Input: part model. Units: mm. Frame: model coordinates. A direction names the side the tool comes from. Round coordinates to 2 decimals unless told otherwise and drop trailing zeros. Loops run counter-clockwise (first coordinate to the right, second up) from the corner with the lowest first, then second, coordinate; pieces in that order, holes last. Notation, with made-up numbers: (42.5, 52.5) -> (65.5, 52.5) arc R15 cw to (65.5, 64.5) -> close; hole circle Ø3 at (26.25, 17.5). An arc over 180 degrees is marked (long way). Answer in a Markdown table with one row per item. Add a question column.
Q1. Section C-C, the plane x = -11. Output: boundary loops of the cut face in (y, z), and give its area (3 significant figures).
Q2. Section D-D, the plane x = -40.5. Output: boundary loops of the cut face in (y, z), and give its area (3 significant figures).
Q3. Section A-A, the plane x = 47.5. Output: boundary loops of the cut face in (y, z), and give its area (3 significant figures).
Q4. Pin query (flat end, axial travel): pin 1 (6.5 mm diameter, centred on x = -28.5, z = 2, fed in from +Y); pin 2 (2.5 mm diameter, centred on y = 4, z = -5, fed in from +X). Return the tip coordinate at first contact, or that it passes through.
Q5. Reachability of faces 1 (the face through (8.25, 4, 0)), 2 (the face through (57.79, 4.39, -6.24)), 3 (the face through (-1, 3, 10.5)), 4 (the face through (-58, 10, 0)), 5 (the face through (-1, 0, -7)) from +Z, -Z, +X, -X, +Y, -Y: full face, straight path, thin tool, end or side. Return the list, or none.
Q6. Mould query, pull axis Z, two halves, no side actions, for faces 6 (the face through (-39.774, 3.944, -2.433)), 7 (the face through (-11.479, 10.859, -9.297)), 8 (the face through (-43, 8, -7)). Classes: pulls with the +Z half, pulls with the -Z half, needs draft (parallel to the pull), parting line crosses it, or undercut.
Q7. Ray query, L1, parallel to X at y = 6.75, z = 0.25; L2, parallel to X at y = 8.5, z = -8.5; L3, parallel to Y at x = 55.25, z = -5. Return the intervals inside material, ascending. Write a range as from..to.
Q8. Section B-B, the plane y = 4. Give the number of separate pieces and of enclosed holes in the cut face, and give its area (3 significant figures).
```python
from build123d import *

# Parameters (mm, degrees)
SKETCH1_W           = 122
SKETCH1_H           = 21
SKETCH1_R           = 8.1
BOSS_EXTRUDE1_DEPTH = 8
CUT_EXTRUDE1_DEPTH  = 122
FILLET2_R           = 1
SKETCH6_W           = 3
SKETCH6_H           = 21
BOSS_EXTRUDE4_DEPTH = 4
FILLET3_R           = 4
SKETCH7_R           = 1.3
CUT_EXTRUDE2_DEPTH  = 10


with BuildPart() as part:
    # Sketch1 → Boss-Extrude1 (new body)
    with BuildSketch(Plane(origin=(0, 0, 0), x_dir=(1, 0, 0), z_dir=(0, 1, 0))):
        Rectangle(SKETCH1_W, SKETCH1_H)
        with Locations((-47.5, 0)):
            Circle(SKETCH1_R, mode=Mode.SUBTRACT)
        with Locations((-23.5, 0)):
            Circle(SKETCH1_R, mode=Mode.SUBTRACT)
        with Locations((23.5, 0)):
            Circle(SKETCH1_R, mode=Mode.SUBTRACT)
        with Locations((47.5, 0)):
            Circle(SKETCH1_R, mode=Mode.SUBTRACT)
    extrude(amount=BOSS_EXTRUDE1_DEPTH)

    # Sketch4 → Cut-Extrude1 (cut)
    with BuildSketch(Plane(origin=(0, 8, 0), x_dir=(1, 0, 0), z_dir=(0, 1, 0))):
        with BuildLine():
            Line((8.25, 4), (4.472135955, 4))
            ThreePointArc((4.472135955, 4), (5.605034154, 2.140932539), (6, 0))
            ThreePointArc((6, 0), (5.605034154, -2.140932539), (4.472135955, -4))
            Line((4.472135955, -4), (8.25, -4))
            Line((8.25, -4), (8.25, 4))
        make_face()
        with BuildLine():
            Line((4.472135955, 4), (-4.472135955, 4))
            ThreePointArc((-4.472135955, 4), (-6, 0), (-4.472135955, -4))
            Line((-4.472135955, -4), (4.472135955, -4))
            ThreePointArc((4.472135955, -4), (5.605034154, -2.140932539), (6, 0))
            ThreePointArc((6, 0), (5.605034154, 2.140932539), (4.472135955, 4))
        make_face()
        with BuildLine():
            ThreePointArc((4.472135955, 4), (0, 6), (-4.472135955, 4))
            Line((-4.472135955, 4), (4.472135955, 4))
        make_face()
        with BuildLine():
            Line((4.472135955, -4), (-4.472135955, -4))
            ThreePointArc((-4.472135955, -4), (0, -6), (4.472135955, -4))
        make_face()
        with BuildLine():
            Line((-4.472135955, 4), (-8.25, 4))
            Line((-8.25, 4), (-8.25, -4))
            Line((-8.25, -4), (-4.472135955, -4))
            ThreePointArc((-4.472135955, -4), (-6, 0), (-4.472135955, 4))
        make_face()
    extrude(amount=-CUT_EXTRUDE1_DEPTH, mode=Mode.SUBTRACT)

    # Fillet2
    fillet2_edges = [part.edges().sort_by_distance(p)[0] for p in [
        (4.472135955, 4, -4),
        (8.25, 4, -4),
        (8.25, 4, 4),
        (4.472135955, 4, 4),
        (-4.472135955, 4, 4),
        (-8.25, 4, 4),
        (-8.25, 4, -4),
        (-4.472135955, 4, -4),
    ]]
    fillet(fillet2_edges, radius=FILLET2_R)

    # Sketch6 → Boss-Extrude4 (add)
    with BuildSketch(Plane(origin=(0, 8, 0), x_dir=(1, 0, 0), z_dir=(0, 1, 0))):
        with Locations((-59.5, 0)):
            Rectangle(SKETCH6_W, SKETCH6_H)
        with Locations((-35.5, 0)):
            Rectangle(SKETCH6_W, SKETCH6_H)
        with Locations((35.5, 0)):
            Rectangle(SKETCH6_W, SKETCH6_H)
        with Locations((59.5, 0)):
            Rectangle(SKETCH6_W, SKETCH6_H)
        with Locations((-11.5, 0)):
            Rectangle(SKETCH6_W, SKETCH6_H)
        with Locations((11.5, 0)):
            Rectangle(SKETCH6_W, SKETCH6_H)
    extrude(amount=BOSS_EXTRUDE4_DEPTH)

    # Fillet3
    fillet3_edges = [part.edges().sort_by_distance(p)[0] for p in [
        (35.5, 12, 10.5),
        (11.5, 12, 10.5),
        (-11.5, 12, 10.5),
        (-35.5, 12, 10.5),
        (35.5, 12, -10.5),
        (11.5, 12, -10.5),
        (-11.5, 12, -10.5),
        (-35.5, 12, -10.5),
    ]]
    fillet(fillet3_edges, radius=FILLET3_R)

    # Sketch7 → Cut-Extrude2 (cut)
    with BuildSketch(Plane(origin=(61, 0, 0), x_dir=(0, 0, -1), z_dir=(1, 0, 0))):
        with Locations((-5, 4)):
            Circle(SKETCH7_R)
        with Locations((5, 4)):
            Circle(SKETCH7_R)
    cut_extrude2 = extrude(amount=-CUT_EXTRUDE2_DEPTH, mode=Mode.SUBTRACT)

    # Mirror1: Cut-Extrude2 across plane
    add(cut_extrude2.mirror(Plane(origin=(0, 0, 0), x_dir=(0, 0, 1), z_dir=(1, 0, 0))), mode=Mode.SUBTRACT)


solid = part.part
```
Answer block:
| question | item | result |
|---|---|---|
| 1 | outline | (0, -10.5) -> (8, -10.5) arc R4 ccw to (12, -6.5) -> (12, 6.5) arc R4 ccw to (8, 10.5) -> (0, 10.5) -> close |
| 1 | area | 245 mm^2 |
| 2 | outline | (0, -10.5) -> (8, -10.5) -> (8, -4.08) -> (0, -4.08) -> close; (0, 4.08) -> (8, 4.08) -> (8, 10.5) -> (0, 10.5) -> close |
| 2 | area | 103 mm^2 |
| 3 | outline | (0, -10.5) -> (8, -10.5) -> (8, -8.1) -> (0, -8.1) -> close; (0, 8.1) -> (8, 8.1) -> (8, 10.5) -> (0, 10.5) -> close |
| 3 | area | 38.4 mm^2 |
| 4 | pin 1 | y = 8 |
| 4 | pin 2 | x = 42.35 |
| 5 | face 1 | +Y, -Y |
| 5 | face 2 | +X |
| 5 | face 3 | +Z, +X, -X, +Y, -Y |
| 5 | face 4 | +Z, -Z, +Y |
| 5 | face 5 | +Z, -Z, +X, -X, -Y |
| 6 | face 6 | undercut |
| 6 | face 7 | pulls with the -Z half |
| 6 | face 8 | needs draft |
| 7 | L1 | -61..-55.6, -39.4..-31.6, -15.4..-8.25, 8.25..15.4, 31.6..39.4, 55.6..61 |
| 7 | L2 | -61..-58, -37..-34, -13..-10, 10..13, 34..37, 58..61 |
| 7 | L3 | 0..2.7, 5.3..8 |
| 8 | separate pieces | 3 |
| 8 | enclosed holes | 3 |
| 8 | area | 1,510 mm^2 |
